Source: CAD feature listing. Evaluate the final solid. Frame: model axes, mm. A direction names the side the tool comes from. Round coordinates to 2 decimals unless told otherwise and drop trailing zeros. Loops run counter-clockwise (first coordinate to the right, second up) from the corner with the lowest first, then second, coordinate; pieces in that order, holes last. Notation, with made-up numbers: (48.25, 12.25) - (106.25, 12.25) arc R24 cw to (106.25, 31.25) - close; hole circle Ø11 at (-24, 73). An arc over 180 degrees is marked (long way). Use CSV: the item, a comma, the result in double quotes. Start each with the question number.
from build123d import *

# Parameters (mm, degrees)
F0_W     = 70.792261
F0_H     = 61.574518
F1_DEPTH = 25.4
F2_R     = 19.369368
F3_DEPTH = 38.1
F4_R     = 13.0339
F5_DEPTH = 38.1


with BuildPart() as f1:
    # F0 (on Front) → F1 (new body)
    with BuildSketch(Plane.XZ):
        with Locations((-1.013951, -3.59492)):
            Rectangle(F0_W, F0_H)
    extrude(amount=F1_DEPTH)

    # F2 (on Front) → F3 (join)
    with BuildSketch(Plane.XZ):
        Circle(F2_R)
    extrude(amount=F3_DEPTH)

    # F4 (on Front) → F5 (cut)
    with BuildSketch(Plane.XZ):
        Circle(F4_R)
    extrude(amount=F5_DEPTH, mode=Mode.SUBTRACT)


solid = f1.part
1. Section query A-A on x = 0. Return the cut outline in (y, z), and give its area (3 significant figures).
2. Section query B-B on z = 0. Return the cut outline in (x, y).
3. Mould query, pull axis X, two halves, no side actions, for faces 1 (the flat face through (-2, -13, -34.382)), 2 (the cylindrical face through (12.04, -18.78, -4.99)), 3 (the cylindrical face through (-15.37, -31.66, -11.79)). Classes: +X half, -X half, draft (parallel to the pull), parting line (faces both ways), or undercut.
4. Contact query for flat-ended pins moving along their axis: P1, Ø1.5, axis at x = 22, z = 2.5, coming from the -Y side; P2, Ø1.5, axis at y = -32.5, z = 5, coming from the +X side; P3, Ø21, axis at x = 0, z = 0, coming from the -Y side. Output: stop coordinate, or through.
5. Line query: line 1 along Z through (x, y) = (0, -17); line 2 along Z through (x, y) = (0, -25.5); line 3 along Y through (x, z) = (-19, 20). Output: solid intervals per line, ascending.
6. Section query C-C on y = -19.5. Return the cut outline in (x, z).
7. Section query D-D on x = 24.5. Return the cut outline in (y, z), and give its area (3 significant figures).
8. Reachability of faces 4 (the flat face through (-17, -25.4, -10)), 5 (the flat face through (4, -38.1, -13)) from +Z, -Z, +X, -X, +Y, -Y: full face, straight path, thin tool, end or side. Return the list, or none.
Values:
1,outline,"(-38.1, -19.37) - (-25.4, -19.37) - (-25.4, -34.38) - (0, -34.38) - (0, -13.03) - (-38.1, -13.03) - close; (-38.1, 13.03) - (0, 13.03) - (0, 27.19) - (-25.4, 27.19) - (-25.4, 19.37) - (-38.1, 19.37) - close"
1,area,"1,060 mm^2"
2,outline,"(-36.41, -25.4) - (-19.37, -25.4) - (-19.37, -38.1) - (-13.03, -38.1) - (-13.03, 0) - (-36.41, 0) - close; (13.03, -38.1) - (19.37, -38.1) - (19.37, -25.4) - (34.38, -25.4) - (34.38, 0) - (13.03, 0) - close"
3,face 1,"draft"
3,face 2,"undercut"
3,face 3,"parting line"
4,P1,"stops at y = -25.4"
4,P2,"stops at x = 18.9"
4,P3,"passes through"
5,line 1,"z = -34.38 to -13.03, 13.03 to 27.19"
5,line 2,"z = -19.37 to -13.03, 13.03 to 19.37"
5,line 3,"y = -25.4 to 0"
6,outline,"(-36.41, -34.38) - (34.38, -34.38) - (34.38, 27.19) - (-36.41, 27.19) - close; hole circle Ø26.07 at (0, 0)"
7,outline,"(-25.4, -34.38) - (0, -34.38) - (0, 27.19) - (-25.4, 27.19) - close"
7,area,"1,560 mm^2"
8,face 4,"-Y"
8,face 5,"+Z, -Z, +X, -X, -Y"
